Verification items for the finished model (mm, model axes). A direction names the side the tool comes from. Coordinates: 2 decimals unless noted, no trailing zeros. Write each loop counter-clockwise with the first axis right and the second up, starting at its lowest first coordinate (ties: lowest second). Pieces come first, ordered by that corner, then holes. Notation, with made-up numbers: (75.25, 42) -> (118.25, 42) arc R29 ccw to (118.25, 71) -> close; hole circle Ø7 at (75.5, -28). An arc over 180 degrees is marked (long way). Answer in a Markdown table with one row per item.
Solid Edge part; units mm, degrees
sketch "Sketch1" plane through (0, 0, 0) normal (0, -1, 0) x (1, 0, 0)
  line L0 (8, 6) -> (-8, 6)
  line L1 (-8, 6) -> (-8, -6)
  line L2 (-8, -6) -> (8, -6)
  line L3 (8, -6) -> (8, 6)
extrude "Protrusion1" add sketch "Sketch1" against normal blind 22
sketch "Sketch2" plane through (0, 0, 0) normal (0, -1, 0) x (1, 0, 0)
  line L0 (6, 4) -> (-6, 4)
  line L1 (-6, 4) -> (-6, -4)
  line L2 (-6, -4) -> (6, -4)
  line L3 (6, -4) -> (6, 4)
extrude "Cutout1" cut sketch "Sketch2" against normal blind 20
sketch "Sketch3" plane through (0, 20, 0) normal (0, -1, 0) x (1, 0, 0)
  line L0 (6, -3) -> (2, -3)
  line L1 (2, -3) -> (2, -4)
  line L2 (2, -4) -> (6, -4)
  line L3 (6, -4) -> (6, -3)
  line L4 (6, 3) -> (2.0028, 3)
  line L5 (2.0028, 3) -> (2.0028, 4)
  line L6 (2.0028, 4) -> (6, 4)
  line L7 (6, 4) -> (6, 3)
extrude "LockSideProtrusion" add sketch "Sketch3" along normal blind 19
sketch "Sketch4" plane through (0, 20, 0) normal (0, -1, 0) x (1, 0, 0)
  line L0 (6, 3) -> (6, -3)
  line L1 (6, -3) -> (2.0028, -3)
  line L2 (2.0028, -3) -> (2.0028, 3)
  line L3 (2.0028, 3) -> (6, 3)
extrude "LockBaseProtrusion" add sketch "Sketch4" along normal blind 2
sketch "Sketch5" plane through (4.0014, 18, 0) normal (0, -1, 0) x (1, 0, 0)
  line L0 (-0.0014, 2.48) -> (-0.0014, -2.48)
  line L1 (-0.0014, -2.48) -> (-2.0014, -2.48)
  line L2 (-2.0014, -2.48) -> (-2.0014, 2.48)
  line L3 (-2.0014, 2.48) -> (-0.0014, 2.48)
extrude "LockProtrusion" add sketch "Sketch5" along normal blind 18.07
sketch "Sketch6" plane through (3, -0.07, 0) normal (0, -1, 0) x (1, 0, 0)
  line L0 (-1, -3.93) -> (-1, 3.93)
  line L1 (-1, 3.93) -> (1, 3.93)
  line L2 (1, 3.93) -> (1, -3.93)
  line L3 (1, -3.93) -> (-1, -3.93)
extrude "LockHeadMainProtrusion" add sketch "Sketch6" along normal blind 3
sketch "Sketch7" plane through (3, -0.07, 0) normal (0, -1, 0) x (1, 0, 0)
  line L0 (-3.4, 3.93) -> (-1, 1.53)
  line L1 (-1, 1.53) -> (-1, 3.93)
  line L2 (-1, 3.93) -> (-3.4, 3.93)
  line L3 (-3.4, -3.93) -> (-1, -1.53)
  line L4 (-1, -1.53) -> (-1, -3.93)
  line L5 (-1, -3.93) -> (-3.4, -3.93)
extrude "LockHeadTriangleProtrusion" add sketch "Sketch7" along normal blind 3
sketch "Sketch8" plane through (1.8, -1.57, -3.93) normal (0, 0, -1) x (1, 0, 0)
  line L0 (-2.2, 1.5) -> (0.2, 1.5)
  line L1 (0.2, 1.5) -> (-2.2, -1.5)
  line L2 (-2.2, -1.5) -> (-2.2, 1.5)
extrude "LockHeadTriangleCut" cut sketch "Sketch8" against normal blind 8.6519
sketch "Sketch9" plane through (4, 7.465, 0) normal (1, 0, 0) x (0, 0, 1)
  line L0 (-3.93, 10.535) -> (3.93, 10.535)
  line L1 (3.93, 10.535) -> (3.93, 8.535)
  line L2 (3.93, 8.535) -> (-3.93, 8.535)
  line L3 (-3.93, 8.535) -> (-3.93, 10.535)
extrude "FlapBaseProtrusion" add sketch "Sketch9" along normal blind 4
sketch "Sketch10" plane through (5, -3.07, 0) normal (0, -1, 0) x (1, 0, 0)
  line L0 (3, 3.93) -> (1, 3.93)
  line L1 (1, 3.93) -> (1, -3.93)
  line L2 (1, -3.93) -> (3, -3.93)
  line L3 (3, -3.93) -> (3, 3.93)
extrude "FlapHandleProtrusion" add sketch "Sketch10" along normal blind 2
fillet "SlotInnerRound" radius 1 3 edges at (0, 0, 4) (-6, 0, 0) (0, 0, -4)
fillet "FlapRound" radius 1 3 edges at (6, -5.07, 0) (8, -5.07, 0) (8, -1.07, 0)
sketch "Sketch11" plane through (4, -3.07, 0) normal (0, -1, 0) x (1, 0, 0)
  line L0 (-1.6753, 0.0864) -> (1.042, 1.2263)
  line L1 (1.042, 1.2263) -> (1.042, -1.1917)
  line L2 (1.042, -1.1917) -> (-1.6753, 0.0864)
extrude "MarkCut" cut sketch "Sketch11" against normal blind 0.8
hole "PushHole" at (-2.0513, 20, 0) direction (0, 1, 0) diameter 4 end through all
fillet "LockTriangleRound" radius 1 2 edges at (2, -1.57, 1.53) (2, -1.57, -1.53)
1. Go/stop test with flat-tipped pins: pin 1 (3 mm diameter, centred on x = -1, z = 0, fed in from +Y); pin 2 (0.5 mm diameter, centred on x = 4.5, z = 3.5, fed in from -Y); pin 3 (0.5 mm diameter, centred on y = -3.5, z = 1.5, fed in from -X); pin 4 (2.5 mm diameter, centred on x = 3.5, y = -3.5, fed in from -Z). Record where each tip stops, or that it passes through.
Findings below:
| item | result |
|---|---|
| pin 1 | stops at y = 22 |
| pin 2 | stops at y = -3.07 |
| pin 3 | stops at x = 6 |
| pin 4 | stops at z = -3.93 |
2. Sectioned sample at A-A, the plane y = 12.25. Record the cut outline in (x, z), and give its area (3 significant figures).
Findings below:
| item | result |
|---|---|
| outline | (-8, -6) -> (8, -6) -> (8, 6) -> (-8, 6) -> close; (2, -2.48) -> (4, -2.48) -> (4, 2.48) -> (2, 2.48) -> close; hole (-6, -4) -> (2, -4) -> (2, -3) -> (6, -3) -> (6, 3) -> (2, 3) -> (2, 4) -> (-6, 4) -> close |
| area | 114 mm² |
3. Access from +Z, -Z, +X, -X, +Y, -Y to the whole of each face (thin tool, end or side, straight path). Record for faces 4 (the face through (2.003, 14.1, 3.3)), 5 (the face through (5, -2, -3.93)), 6 (the face through (0.1, 22, 0.1)), 7 (the face through (-1, 10, -4)), 8 (the face through (0, 11, -6)).
Findings below:
| item | result |
|---|---|
| face 4 | none |
| face 5 | -Z, +X, -X, -Y |
| face 6 | +Z, -Z, +X, -X, +Y |
| face 7 | -Y |
| face 8 | -Z, +X, -X, +Y, -Y |
4. Material ranges on probe 1 along X at (y, z) = (9.75, -2); probe 2 along X at (y, z) = (20.9, 0); probe 3 along Z at (x, y) = (-0.5, 14.5), recorded low to high. Write a range as from..to.
Findings below:
| item | result |
|---|---|
| probe 1 | x = -8..-6, 2..4, 6..8 |
| probe 2 | x = -8..-4.05, -0.05..8 |
| probe 3 | z = -6..-4, 4..6 |
5. Sectioned sample at D-D, the plane x = -6.5. Record the cut outline in (y, z).
Findings below:
| item | result |
|---|---|
| outline | (0, -6) -> (22, -6) -> (22, 6) -> (0, 6) -> (0, 5) arc R1 ccw to (0.13, 4.5) -> (0.13, -4.5) arc R1 ccw to (0, -5) -> close |
6. Release check for a two-part mould opening along Y. For faces 1 (the face through (5, -2, 3.93)), 2 (the face through (1.35, -2.26, 3.13)), 3 (the face through (6, 9, 0)) record: released by +Y, released by -Y, zero draft, split by the parting line, or undercut.
Findings below:
| item | result |
|---|---|
| face 1 | zero draft |
| face 2 | released by -Y |
| face 3 | undercut |
7. Sectioned sample at B-B, the plane x = 0.75. Record the cut outline in (y, z).
Findings below:
| item | result |
|---|---|
| outline | (-1.51, -3.93) -> (-0.07, -3.93) -> (-0.07, -2.78) -> (-1.51, -2.78) -> close; (-1.51, 2.78) -> (-0.07, 2.78) -> (-0.07, 3.93) -> (-1.51, 3.93) -> close; (0, -6) -> (22, -6) -> (22, 6) -> (0, 6) -> (0, 5) arc R1 ccw to (1, 4) -> (20, 4) -> (20, -4) -> (1, -4) arc R1 ccw to (0, -5) -> close |
